Verification items for the finished model (mm, model axes). Round coordinates to 2 decimals unless told otherwise and drop trailing zeros. Use one line per item in the form item = value. Start each with the question number.
Item 1: Release check for a two-part mould opening along Y. For faces 1 (the conical face through (-25.8, -26.3, 20.1)), 2 (the conical face through (45.973, 32.817, -10.335)), 3 (the conical face through (25.76, 56.83, -44.4)), 4 (the flat face through (-50.8, 6, 39)) record: +Y half, -Y half, draft (parallel to the pull), parting line (faces both ways), or undercut.
Item 2: Thickness scan on probe 1 along Z at (x, y) = (2, 15.5); probe 2 along Y at (x, z) = (-27, -18); probe 3 along Z at (x, y) = (-24.5, -1.5). Record the ranges inside material, lowest first. Write a range as [from, to].
Item 3: Go/stop test with flat-tipped pins: pin 1 Ø2 at (x, z) = (26.5, -5) entering from -Y; pin 2 Ø6 at (x, z) = (-4.5, 15.5) entering from +Y; pin 3 Ø2 at (x, z) = (-40.5, 14.5) entering from +Y. Record where each tip stops, or that it passes through.
from build123d import *

# Parameters (mm, degrees)
F0_R     = 31.75
F1_DEPTH = 50.8
F1_TAPER = 3
F2_SIZE  = 25.4
F3_SIZE  = 5.08


with BuildPart() as f1:
    # F0 (on Right) → F1 (new body, symmetric)
    with BuildSketch(Plane.YZ):
        with BuildLine():
            Line((63.5, 76.2), (-25.4, 76.2))
            ThreePointArc((-25.4, 76.2), (-43.3605122421, 68.7605122421), (-50.8, 50.8))
            Line((-50.8, 50.8), (-50.8, -50.8))
            Line((-50.8, -50.8), (44.45, -50.8))
            ThreePointArc((44.45, -50.8), (57.9203841816, -45.2203841816), (63.5, -31.75))
            Line((63.5, -31.75), (63.5, 76.2))
        make_face()
        Circle(F0_R, mode=Mode.SUBTRACT)
    extrude(amount=F1_DEPTH, both=True, taper=F1_TAPER)

    # F2
    f2_edges = [f1.edges().sort_by_distance(p)[0] for p in [
        (25.4, 62.168842, 74.868842),
        (-25.4, 62.168842, 74.868842),
    ]]
    chamfer(f2_edges, length=F2_SIZE)

    # F3
    f3_edges = [f1.edges().sort_by_distance(p)[0] for p in [
        (50.8, -34.412315, 0),
    ]]
    chamfer(f3_edges, length=F3_SIZE)


solid = f1.part
Output values:
q1.face_1 = undercut
q1.face_2 = undercut
q1.face_3 = +Y half
q1.face_4 = draft
q2.probe_1 = [-50.7, -27.83], [27.83, 76.1]
q2.probe_2 = [-49.38, -27.86], [27.86, 62.08]
q2.probe_3 = [-49.52, -33], [33, 74.92]
q3.pin_1 = -49.46
q3.pin_2 = 63.42
q3.pin_3 = 61.43
